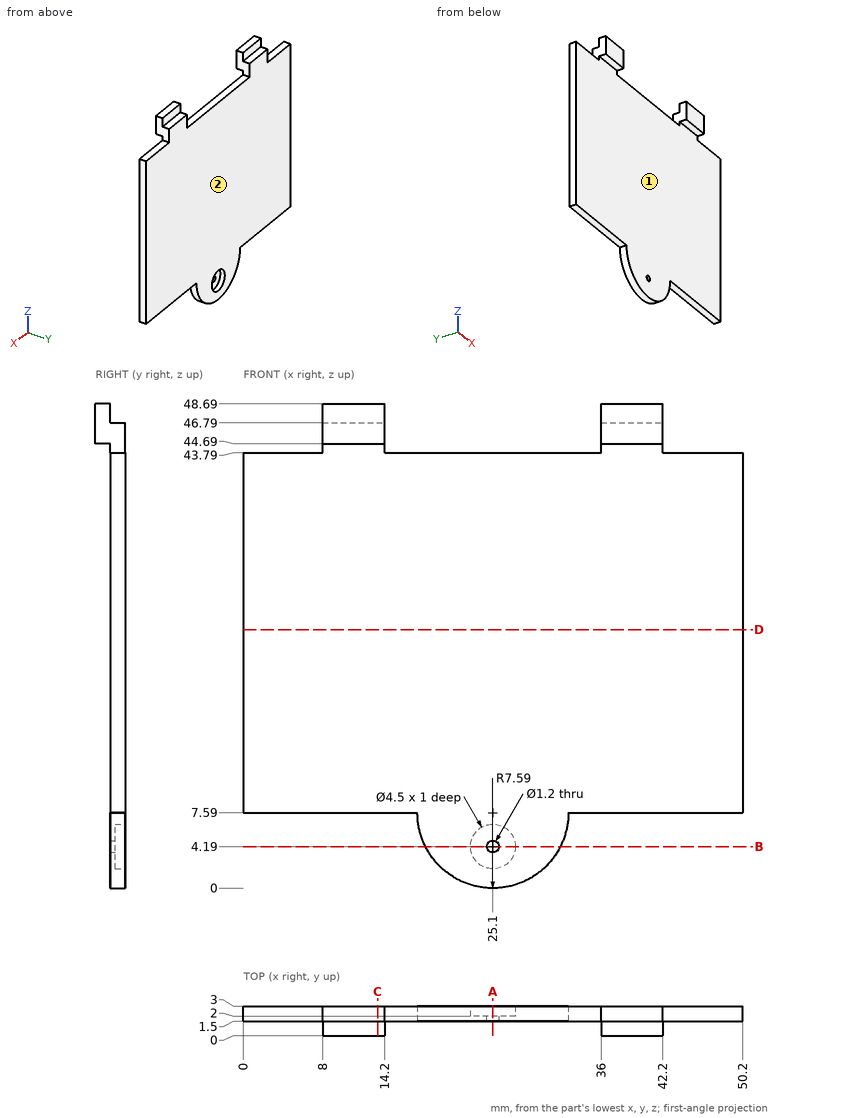
The drawing under review shows one solid part. Ordinate dimensions are in mm from its lowest x, y, z. A direction names the side the tool comes from. Round coordinates to 2 decimals unless told otherwise and drop trailing zeros. Loops run counter-clockwise (first coordinate to the right, second up) from the corner with the lowest first, then second, coordinate; pieces in that order, holes last. Notation, with made-up numbers: (54.25, 65.25) -> (106.25, 65.25) arc R29 cw to (106.25, 93.25) -> close; hole circle Ø4 at (-36, 86). An arc over 180 degrees is marked (long way). Answer in a Markdown table with one row per item.
1) For pin 1 Ø1.6 at (x, z) = (25.1, 4.19) entering from -Y; pin 2 Ø0.6 at (x, z) = (12.5, 48) entering from +Y; pin 3 Ø0.9 at (y, z) = (2, 46) entering from -X; pin 4 Ø1.5 at (x, z) = (40.5, 47.5) entering from +Y, all flat-tipped, find the tip position at first contact; note any pin that passes through.
Taken from the geometry:
| item | result |
|---|---|
| pin 1 | stops at y = 1.5 |
| pin 2 | stops at y = 1.5 |
| pin 3 | stops at x = 8 |
| pin 4 | stops at y = 3 |
2) Consider section A-A, the plane x = 25.1. Write out the cut boundary in (y, z), plus the area to 3 significant figures.
Taken from the geometry:
| item | result |
|---|---|
| outline | (1.5, 0) -> (3, 0) -> (3, 1.94) -> (2, 1.94) -> (2, 3.59) -> (1.5, 3.59) -> close; (1.5, 4.79) -> (2, 4.79) -> (2, 6.44) -> (3, 6.44) -> (3, 43.79) -> (1.5, 43.79) -> close |
| area | 60.6 mm² |
3) Wall thickness on line 1 along X through (y, z) = (1.6, 44.5); line 2 along Z through (x, y) = (25.1, 1.6); line 3 along Z through (x, y) = (25.1, 2.8): over which ranges is each line inside the solid? List them lowest first.
Taken from the geometry:
| item | result |
|---|---|
| line 1 | x = 8 to 14.2, 36 to 42.2 |
| line 2 | z = 0 to 3.59, 4.79 to 43.79 |
| line 3 | z = 0 to 1.94, 6.44 to 43.79 |
4) Consider section B-B, the plane z = 4.19. Write out the cut boundary in (x, y), plus the area to 3 significant figures.
Taken from the geometry:
| item | result |
|---|---|
| outline | (18.31, 1.5) -> (24.5, 1.5) -> (24.5, 2) -> (22.85, 2) -> (22.85, 3) -> (18.31, 3) -> close; (25.7, 1.5) -> (31.89, 1.5) -> (31.89, 3) -> (27.35, 3) -> (27.35, 2) -> (25.7, 2) -> close |
| area | 15.3 mm² |
5) Tool access review of the marked faces 1 and 2: name each direction out of +Z, -Z, +X, -X, +Y, -Y from which nothing blocks a thin tool from reaching the whole face with its end or side.
Taken from the geometry:
| item | result |
|---|---|
| face 1 | -Z, +X, -X, -Y |
| face 2 | +Z, -Z, +X, -X, +Y |
6) Consider section D-D, the plane z = 26. Write out the cut boundary in (x, y), plus the area to 3 significant figures.
Taken from the geometry:
| item | result |
|---|---|
| outline | (0, 1.5) -> (50.2, 1.5) -> (50.2, 3) -> (0, 3) -> close |
| area | 75.3 mm² |
7) Consider section C-C, the plane x = 13.5. Write out the cut boundary in (y, z).
Taken from the geometry:
| item | result |
|---|---|
| outline | (0, 44.69) -> (1.5, 44.69) -> (1.5, 7.59) -> (3, 7.59) -> (3, 46.79) -> (1.5, 46.79) -> (1.5, 48.69) -> (0, 48.69) -> close |
